CAD build for the part. Positions are in the model's coordinates, mm. Face numbers are marked on the shaded views. A direction names the side the tool comes from. Round coordinates to 2 decimals unless told otherwise and drop trailing zeros. Write each loop counter-clockwise with the first axis right and the second up, starting at its lowest first coordinate (ties: lowest second). Pieces come first, ordered by that corner, then holes. Notation, with made-up numbers: (66, 71.25) -> (103, 71.25) arc R28 cw to (103, 109.25) -> close; hole circle Ø10 at (-2, -19). An arc over 180 degrees is marked (long way). Put each result on its own line as item: value. Start each with the question number.
1. Saw through at C-C on z = 11. List the corners of the cut face in (x, y).
2. Flat gauge pins, fed straight in: P1, Ø3, axis at y = 0, z = 11, coming from the +X side; P2, Ø8, axis at x = -7.5, y = 1, coming from the +Z side; P3, Ø4, axis at y = -2.5, z = 3, coming from the +X side; P4, Ø5, axis at y = 3, z = 2, coming from the -X side. Where does each tip first touch, or does it go through?
3. Pull direction Y, two halves, no side cores. Call the marked faces 1, 2 and 3: pulls with the +Y half, pulls with the -Y half, needs draft (parallel to the pull), parting line crosses it, or undercut.
4. Saw through at A-A on y = 0. List the corners of the cut face in (x, z).
5. Drill centre lines: line 1 (Y direction, x = 0, z = 2.7); line 2 (X direction, y = 3, z = 5); line 3 (X direction, y = -13.05, z = 11). Where is each one in solid material? Low to high. Write a range as from..to.
6. 3-axis set-ups, long thin cutter, end or side, ignore diameter. For the marked faces 4, 5 and 6: which of +Z, -Z, +X, -X, +Y, -Y reach the whole face in a straight line?
7. Saw through at D-D on z = 8. List the corners of the cut face in (x, y), and give its area (3 significant figures).
from build123d import *

# Parameters (mm, degrees)
SKETCH_1_R               = 17.5
EXTRUDE_1_DEPTH          = 16
HOLE_WIZARD_M27_1_D      = 24
HOLE_WIZARD_M27_1_DEPTH  = 9
HOLE_WIZARD_M27_1_TIP    = 6.92820323
SKETCH_4_R               = 17.5
EXTRUDE_2_DEPTH          = 4
SKETCH_5_W               = 3
SKETCH_5_H               = 10
SKETCH_6_R               = 2
CUT_EXTRUDE_1_DEPTH      = 30.470324057
PATTERN_CIRCULAR_1_COUNT = 4
SKETCH_7_R               = 8
CUT_EXTRUDE_2_DEPTH      = 30.47032423
CHAMFER_1_SIZE           = 2


with BuildPart() as part:
    # 草图1 → 凸台-拉伸1 (new body)
    with BuildSketch(Plane.XY):
        Circle(SKETCH_1_R)
    extrude(amount=EXTRUDE_1_DEPTH)

    # M27 螺纹孔1
    with Locations(Plane.XY.offset(16)):
        with Locations((0, 0)):
            Hole(HOLE_WIZARD_M27_1_D / 2, depth=HOLE_WIZARD_M27_1_DEPTH)
            with Locations((0, 0, -(HOLE_WIZARD_M27_1_DEPTH + HOLE_WIZARD_M27_1_TIP / 2))):  # 120° drill point
                Cone(0, HOLE_WIZARD_M27_1_D / 2, HOLE_WIZARD_M27_1_TIP, mode=Mode.SUBTRACT)

    # 草图4 → 凸台-拉伸2 (add)
    with BuildSketch(Plane(origin=(0, 0, 0), x_dir=(-1, 0, 0), z_dir=(0, 0, -1))):
        with Locations(Location((0, 0, 0), (0, 0, 180))):
            Circle(SKETCH_4_R)
    extrude_2 = extrude(amount=-EXTRUDE_2_DEPTH)

    # 草图5 → 切除-旋转1 (revolve, cut)
    with BuildSketch(Plane(origin=(0, 0, 0), x_dir=(0, 0, -1), z_dir=(1, 0, 0)), mode=Mode.PRIVATE) as cut_revolve_1_sk:
        with Locations((-5.5, 9.5)):
            Rectangle(SKETCH_5_W, SKETCH_5_H)
    revolve(cut_revolve_1_sk.sketch.rotate(Axis((0, 0, 16), (0, 0, -1)), 90), axis=Axis((0, 0, 16), (0, 0, -1)), mode=Mode.SUBTRACT)

    # 草图6 → 切除-拉伸1 (cut, through all)
    with BuildSketch(Plane(origin=(0, 0, 0), x_dir=(0, 0, -1), z_dir=(1, 0, 0))):
        with Locations((-11, 0)):
            Circle(SKETCH_6_R)
    cut_extrude_1 = extrude(amount=-CUT_EXTRUDE_1_DEPTH, mode=Mode.SUBTRACT)

    # 阵列(圆周)1: 凸台-拉伸2, 切除-拉伸1 ×4 about axis
    pattern_circular_1_axis = Axis((0, 0, 16), (0, 0, -1))
    add([extrude_2.rotate(pattern_circular_1_axis, i * 360 / PATTERN_CIRCULAR_1_COUNT) for i in range(1, PATTERN_CIRCULAR_1_COUNT)])
    add([cut_extrude_1.rotate(pattern_circular_1_axis, i * 360 / PATTERN_CIRCULAR_1_COUNT) for i in range(1, PATTERN_CIRCULAR_1_COUNT)], mode=Mode.SUBTRACT)

    # 草图7 → 切除-拉伸2 (cut, through all)
    with BuildSketch(Plane(origin=(0, 0, 0), x_dir=(-1, 0, 0), z_dir=(0, 0, -1))):
        Circle(SKETCH_7_R)
    extrude(amount=-CUT_EXTRUDE_2_DEPTH, mode=Mode.SUBTRACT)

    # 倒角1
    chamfer_1_edges = [part.edges().sort_by_distance(p)[0] for p in [
        (-17.5, 0, 0),
        (-17.5, 0, 16),
    ]]
    chamfer(chamfer_1_edges, length=CHAMFER_1_SIZE)


solid = part.part
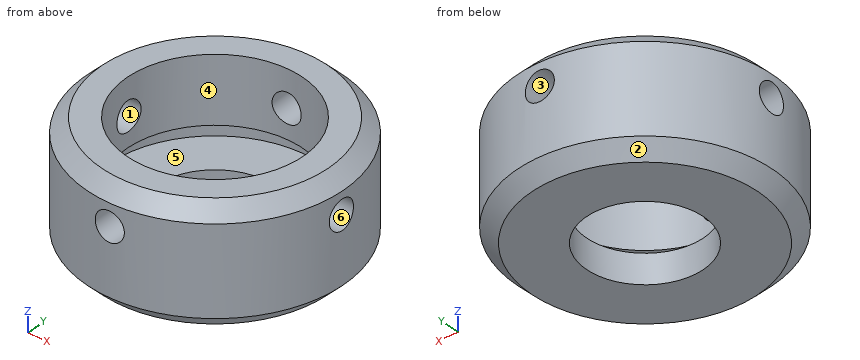
Return value:
1. outline: (-17.39, -2) arc R17.5 ccw to (-2, -17.39) -> (-2, -11.83) arc R12 cw to (-11.83, -2) -> close; (-17.39, 2) -> (-11.83, 2) arc R12 cw to (-2, 11.83) -> (-2, 17.39) arc R17.5 ccw to start; (2, -17.39) arc R17.5 ccw to (17.39, -2) -> (11.83, -2) arc R12 cw to (2, -11.83) -> close; (2, 11.83) arc R12 cw to (11.83, 2) -> (17.39, 2) arc R17.5 ccw to (2, 17.39) -> close
2. P1: passes through
2. P2: stops at z = 4
2. P3: stops at x = 17.49
2. P4: stops at x = -17.49
3. face 1: undercut
3. face 2: parting line crosses it
3. face 3: needs draft
4. outline: (-17.5, 2) -> (-15.5, 0) -> (-8, 0) -> (-8, 4) -> (-14.5, 4) -> (-14.5, 7) -> (-12, 7) -> (-12, 9) -> (-17.5, 9) -> close; (-17.5, 13) -> (-12, 13) -> (-12, 16) -> (-15.5, 16) -> (-17.5, 14) -> close; (8, 0) -> (15.5, 0) -> (17.5, 2) -> (17.5, 9) -> (12, 9) -> (12, 7) -> (14.5, 7) -> (14.5, 4) -> (8, 4) -> close; (12, 13) -> (17.5, 13) -> (17.5, 14) -> (15.5, 16) -> (12, 16) -> close
5. line 1: y = -17.5..-8, 8..17.5
5. line 2: x = -17.24..-14.19, 14.19..17.24
5. line 3: x = -11.66..-2, 2..11.66
6. face 4: +Z
6. face 5: none
6. face 6: +X, -X
7. outline: circle Ø35 at (0, 0); hole circle Ø24 at (0, 0)
7. area: 510 mm^2
